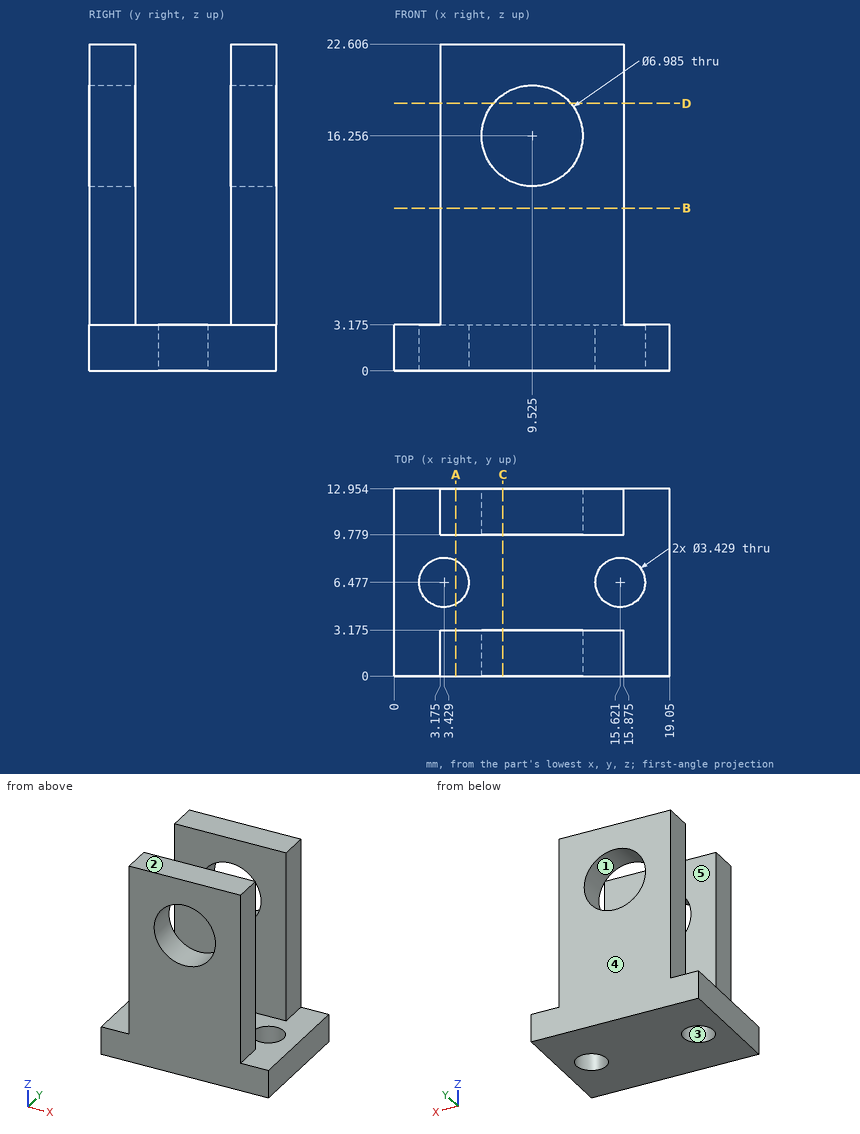
Answer from the drawing. Dimensions are ordinates in mm from the lowest x, y and z of the part. A direction names the side the tool comes from. Give positions to 0.01 mm unless a question says otherwise; leave off trailing zeros. Loops run counter-clockwise (first coordinate to the right, second up) from the corner with the lowest first, then second, coordinate; pieces in that order, holes last.
Item 1: The part is cut by section A-A (x = 4.25). Write down the section's boundary in (y, z) (3 decimals).
Item 2: Each of these flat-tipped pins is pushed along its axis until it touches: pin 1 Ø3.5 at (y, z) = (1.5, 17.5) entering from -X (3 decimals); pin 2 Ø4 at (y, z) = (4, 16) entering from +X (3 decimals). Where does it stop, or does it pass through?
Item 3: The part is cut by section C-C (x = 7.5). Write down the section's boundary in (y, z) (3 decimals), and give its area (3 significant figures).
Item 4: The mould has two halves that part along Z. Classify the marked faces 1, 2 and 3: released by +Z, released by -Z, zero draft, split by the parting line, or undercut.
Item 5: The part is cut by section B-B (z = 11.25). Write down the section's boundary in (x, y) (3 decimals).
Item 6: The part is cut by section D-D (z = 18.5). Write down the section's boundary in (x, y) (3 decimals).
Item 7: Find the intervals of material crossed by line 1 along Y through (x, z) = (6, 17.25) (3 decimals); line 2 along X through (y, z) = (12, 11.5) (3 decimals); line 3 along Z through (x, y) = (8.5, 2.25), in increasing order.
Item 8: For the marked faces 4 and 5, determine the directions among +Z, -Z, +X, -X, +Y, -Y from which every point of the face is accessible in a straight line to the end or side of a thin tool.
Taken from the geometry:
1. outline: (0, 0) - (4.972, 0) - (4.972, 3.175) - (3.175, 3.175) - (3.175, 22.606) - (0, 22.606) - close; (7.982, 0) - (12.954, 0) - (12.954, 22.606) - (9.779, 22.606) - (9.779, 3.175) - (7.982, 3.175) - close
2. pin 1: stops at x = 3.175
2. pin 2: stops at x = 15.875
3. outline: (0, 0) - (12.954, 0) - (12.954, 13.41) - (9.779, 13.41) - (9.779, 3.175) - (3.175, 3.175) - (3.175, 13.41) - (0, 13.41) - close; (0, 19.102) - (3.175, 19.102) - (3.175, 22.606) - (0, 22.606) - close; (9.779, 19.102) - (12.954, 19.102) - (12.954, 22.606) - (9.779, 22.606) - close
3. area: 128 mm2
4. face 1: undercut
4. face 2: released by +Z
4. face 3: zero draft
5. outline: (3.175, 0) - (15.875, 0) - (15.875, 3.175) - (3.175, 3.175) - close; (3.175, 9.779) - (15.875, 9.779) - (15.875, 12.954) - (3.175, 12.954) - close
6. outline: (3.175, 0) - (6.849, 0) - (6.849, 3.175) - (3.175, 3.175) - close; (3.175, 9.779) - (6.849, 9.779) - (6.849, 12.954) - (3.175, 12.954) - close; (12.201, 0) - (15.875, 0) - (15.875, 3.175) - (12.201, 3.175) - close; (12.201, 9.779) - (15.875, 9.779) - (15.875, 12.954) - (12.201, 12.954) - close
7. line 1: y = 0 to 3.175, 9.779 to 12.954
7. line 2: x = 3.175 to 15.875
7. line 3: z = 0 to 12.92, 19.59 to 22.61
8. face 4: +Z, -Z, +X, -X, +Y
8. face 5: +Z, +X, -X
